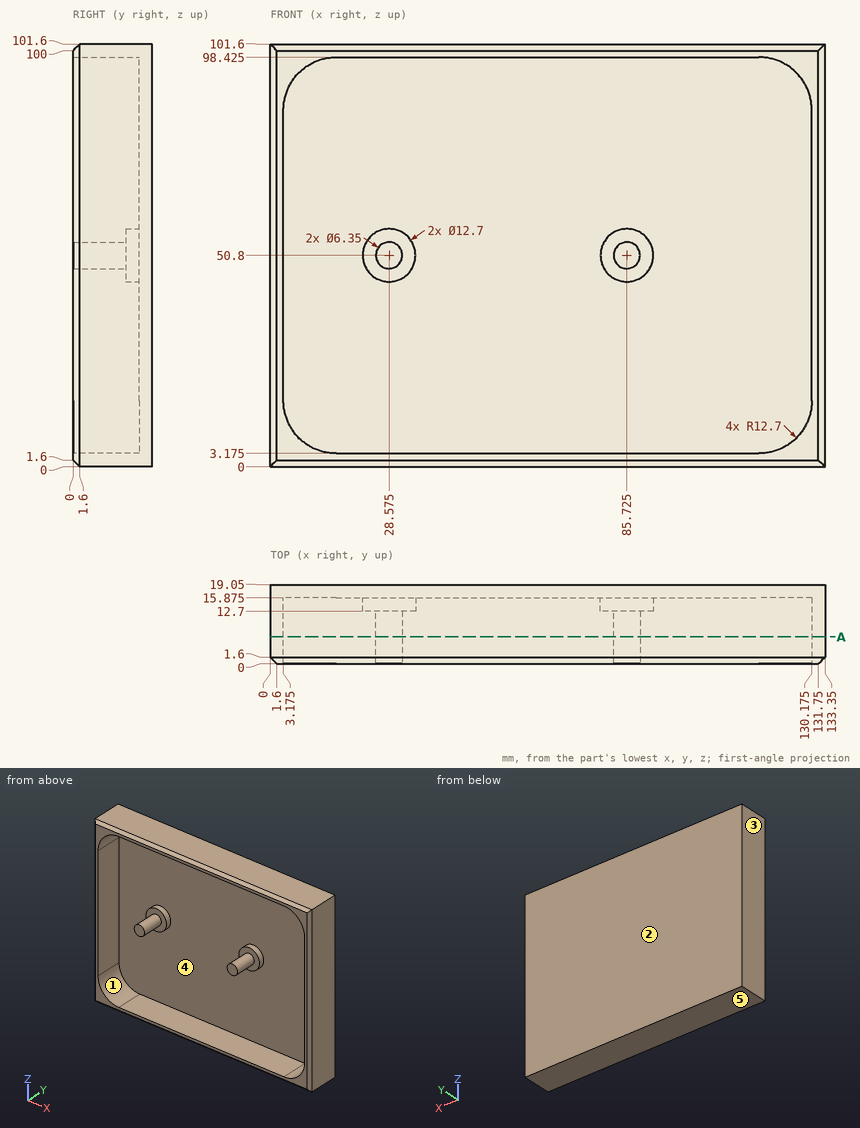
For this review, use the dimensioned drawing (mm, ordinates from the lowest corner) and the shaded views. A direction names the side the tool comes from. Round coordinates to 2 decimals unless told otherwise and drop trailing zeros. Loops run counter-clockwise (first coordinate to the right, second up) from the corner with the lowest first, then second, coordinate; pieces in that order, holes last. Notation, with made-up numbers: M -21,-21 L 28,-21 A14 cw 28,4 Z; hole C 63.5,35 d2. An arc over 180 degrees is marked long. Answer as a JSON object with one key per item and string values.
(1) Tool access review of the marked faces 1 and 2: name each direction out of +Z, -Z, +X, -X, +Y, -Y from which nothing blocks a thin tool from reaching the whole face with its end or side.
Resolved:
{"face 1": "-Y", "face 2": "+Z, -Z, +X, -X, +Y"}
(2) Take a section at A-A on y = 6.5. Give the boundary of the cut face in (x, z) (3 decimals).
Resolved:
{"outline": "M 0,0 L 133.35,0 L 133.35,101.6 L 0,101.6 Z; C 28.575,50.8 d6.35; C 85.725,50.8 d6.35; hole M 3.175,15.875 A12.7 ccw 15.875,3.175 L 117.475,3.175 A12.7 ccw 130.175,15.875 L 130.175,85.725 A12.7 ccw 117.475,98.425 L 15.875,98.425 A12.7 ccw 3.175,85.725 Z"}
(3) Clearance check with a flat-ended pin moving along its axis: P1, Ø6, axis at x = 83, z = 27.5, coming from the -Y side (3 decimals). State where the tip first meets the part, or that it passes through.
Resolved:
{"P1": "y = 15.875"}
(4) To check wall thickness, follow line 1 along X through (y, z) = (8.25, 22.5) (3 decimals); line 2 along Z through (x, y) = (80, 4.75) (3 decimals); line 3 along Z through (x, y) = (87, 3) (1 decimal). State the ranges of each line that lie inside material, in increasing order.
Resolved:
{"line 1": "0 to 3.175, 130.175 to 133.35", "line 2": "0 to 3.175, 98.425 to 101.6", "line 3": "0 to 3.2, 47.9 to 53.7, 98.4 to 101.6"}
(5) Draft analysis for pull direction X (two halves, no side actions). For the marked faces 3, 4 and 5, state which applies: released by +X, released by -X, zero draft, split by the parting line, or undercut.
Resolved:
{"face 3": "released by -X", "face 4": "undercut", "face 5": "zero draft"}
